Geometry: final body of the model. Coordinates: model frame, mm. A direction names the side the tool comes from. Give positions to 0.01 mm unless a question says otherwise; leave off trailing zeros. Loops run counter-clockwise (first coordinate to the right, second up) from the corner with the lowest first, then second, coordinate; pieces in that order, holes last.
from build123d import *

# Parameters (mm, degrees)
SKETCH1_R               = 4
SKETCH1_R_2             = 2
BOSS_EXTRUDE1_DEPTH     = 10
SKETCH3_W               = 31.19
SKETCH3_H               = 12
CUT_EXTRUDE1_DEPTH      = 20
DRAFT1_ANGLE            = 5.03318731
CUT_EXTRUDE2_DEPTH      = 99.920109305
CUT_EXTRUDE2_DEPTH_BACK = 99.920109305
SKETCH4_W               = 26
SKETCH4_H               = 12


with BuildPart() as part:
    # Sketch1 → Boss-Extrude1 (new, symmetric)
    with BuildSketch(Plane(origin=(0, 0, 0), x_dir=(1, 0, 0), z_dir=(0, 1, 0))):
        with BuildLine():
            Line((0, 18.805), (0, -18.805))
            Line((0, -18.805), (-86.1, -10.5))
            ThreePointArc((-86.1, -10.5), (-96.6, 0), (-86.1, 10.5))
            Line((-86.1, 10.5), (0, 18.805))
        make_face()
        with Locations(Location((-86.1, 0, 0), (0, 0, 270))):
            Circle(SKETCH1_R, mode=Mode.SUBTRACT)
        with Locations(Location((-5.1, 6.005, 0), (0, 0, 270))):
            Circle(SKETCH1_R_2, mode=Mode.SUBTRACT)
        with Locations(Location((-5.1, -6.005, 0), (0, 0, 270))):
            Circle(SKETCH1_R_2, mode=Mode.SUBTRACT)
    extrude(amount=BOSS_EXTRUDE1_DEPTH, both=True)

    # Sketch3 → Cut-Extrude1 (cut)
    with BuildSketch(Plane(origin=(0, 0, 0), x_dir=(0, 0, -1), z_dir=(1, 0, 0))):
        Rectangle(SKETCH3_W, SKETCH3_H)
    extrude(amount=-CUT_EXTRUDE1_DEPTH, mode=Mode.SUBTRACT)

    # Draft1
    draft1_faces = [part.faces().sort_by_distance(p)[0] for p in [
        (-10, 0, 15.595),
        (-10, 0, -15.595),
    ]]
    draft(draft1_faces, Plane(origin=(0, 10, -18.805), x_dir=(0, 0, 1), z_dir=(1, 0, 0)), DRAFT1_ANGLE)

    # Sketch4 → Cut-Extrude2 (cut, two sides: drawn at the far end of the back side and taken through both)
    with BuildSketch(Plane.XY.offset(-CUT_EXTRUDE2_DEPTH_BACK)):
        with Locations((-83.6, 0)):
            Rectangle(SKETCH4_W, SKETCH4_H)
    extrude(amount=CUT_EXTRUDE2_DEPTH + CUT_EXTRUDE2_DEPTH_BACK, mode=Mode.SUBTRACT)


solid = part.part
Item 1: Section query A-A on z = 0. Return loops of the section in (x, y).
Values follow:
outline: (-96.6, -10) - (-90.1, -10) - (-90.1, -6) - (-96.6, -6) - close; (-96.6, 6) - (-90.1, 6) - (-90.1, 10) - (-96.6, 10) - close; (-82.1, -10) - (0, -10) - (0, -6) - (-20, -6) - (-20, 6) - (0, 6) - (0, 10) - (-82.1, 10) - (-82.1, 6) - (-70.6, 6) - (-70.6, -6) - (-82.1, -6) - close
Item 2: Section query D-D on y = -2.25. Return loops of the section in (x, z) (3 decimals), plus the area to 3 significant figures.
Values follow:
outline: (-70.6, -11.995) - (0, -18.805) - (0, -15.595) - (-20, -13.834) - (-20, 13.834) - (0, 15.595) - (0, 18.805) - (-70.6, 11.995) - close
area: 1,590 mm2
Item 3: Pin query (flat end, axial travel): pin 1 (5 mm diameter, centred on x = -86.1, z = 0, fed in from -Y); pin 2 (6 mm diameter, centred on y = 2, z = -3.5, fed in from +X); pin 3 (1 mm diameter, centred on y = 0, z = -2.5, fed in from -X); pin 4 (6 mm diameter, centred on x = -17, y = -1, fed in from -Z). Return the tip coordinate at first contact, or that it passes through.
Values follow:
pin 1: passes through
pin 2: stops at x = -20
pin 3: stops at x = -70.6
pin 4: stops at z = -17.45
Item 4: Draft query along X for faces 4 (the face through (-43.653, 0.14, -14.594)), 5 (the face through (-4.499, -8.028, 7.913)), 6 (the face through (-10, -6, 0)). Return one class per face: +X half, -X half, draft (parallel to the pull), parting line (faces both ways), or undercut.
Values follow:
face 4: -X half
face 5: undercut
face 6: draft
Item 5: Ray query, probe 1 along Z at (x, y) = (-5.1, -7.8) (3 decimals); probe 2 along Y at (x, z) = (-74, 2); probe 3 along Z at (x, y) = (-86.1, -7.1). Return the intervals inside material, ascending.
Values follow:
probe 1: z = -18.313 to -8.005, -4.005 to 4.005, 8.005 to 18.313
probe 2: y = -10 to -6, 6 to 10
probe 3: z = -10.5 to -4, 4 to 10.5
Item 6: Section query C-C on x = -5.1. Return loops of the section in (y, z) (3 decimals).
Values follow:
outline: (-10, -18.313) - (10, -18.313) - (10, -8.005) - (6, -8.005) - (6, -15.146) - (-6, -15.146) - (-6, -8.005) - (-10, -8.005) - close; (-10, -4.005) - (-6, -4.005) - (-6, 4.005) - (-10, 4.005) - close; (-10, 8.005) - (-6, 8.005) - (-6, 15.146) - (6, 15.146) - (6, 8.005) - (10, 8.005) - (10, 18.313) - (-10, 18.313) - close; (6, -4.005) - (10, -4.005) - (10, 4.005) - (6, 4.005) - close
Item 7: Set-up query: faces 1 (the face through (-10, 6, 0)), 2 (the face through (-48, 10, 0)), 3 (the face through (-70.6, 0, 0)). Return all of +Z, -Z, +X, -X, +Y, -Y with unobstructed straight access to the full face (end or side cutting, diameter ignored); none if empty.
Values follow:
face 1: +X
face 2: +Z, -Z, +X, -X, +Y
face 3: +Z, -Z, -X
Item 8: Section query B-B on y = 8. Return loops of the section in (x, z) (3 decimals).
Values follow:
outline: (-86.1, -10.5) - (0, -18.805) - (0, 18.805) - (-86.1, 10.5) arc R10.5 ccw to start; hole circle Ø8 at (-86.1, 0); hole circle Ø4 at (-5.1, -6.005); hole circle Ø4 at (-5.1, 6.005)
